Geometry check sheet. Reference: the model listing, model coordinates, mm. Face numbers are marked on the shaded views. A direction names the side the tool comes from. Round coordinates to 2 decimals unless told otherwise and drop trailing zeros. Order: outer loops, then holes, each group sorted by start corner. A loop starts at its lowest first (then second) coordinate and runs counter-clockwise, first axis right, second up. Notation, with made-up numbers: (73.5, 2.5) - (128.5, 2.5) arc R19 ccw to (128.5, 35.5) - close; hole circle Ø1 at (29, 42.5). An arc over 180 degrees is marked (long way). One line per question, with ' | ' between items. Start each with the question number.
Q1. Sectioned sample at B-B, the plane z = 12.5. Enter the section's corners in (x, y), then the cut area to 4 significant figures.
Q2. Gauge pin test, flat ends, axial feed: P1, Ø8, axis at x = 25, y = 17.5, coming from the -Z side; P2, Ø2.5, axis at x = 2, z = 25.5, coming from the +Y side; P3, Ø5, axis at x = 8, z = 18.5, coming from the +Y side; P4, Ø0.9, axis at x = 43.5, z = 16, coming from the +Y side. Record the tip position at first contact, or that the pin passes through.
Q3. Mould release check, pull along Z, two halves, no side actions. Record for the marked faces 3, 4, 5 and 6: +Z half, -Z half, draft (parallel to the pull), parting line (faces both ways), or undercut.
Q4. Sectioned sample at A-A, the plane y = 5.5. Enter the section's corners in (x, z).
Q5. Sectioned sample at C-C, the plane x = 7. Enter the section's corners in (y, z), then the cut area to 4 significant figures.
Q6. Sectioned sample at D-D, the plane z = 1. Enter the section's corners in (x, y).
Q7. Tool access check on the marked faces 1 and 2. Record the directions out of +Z, -Z, +X, -X, +Y, -Y that give a thin tool (end or side, any length) a straight path to the whole face; none if there is none.
Q8. Material ranges on line 1 along X through (y, z) = (12.5, 32.5); line 2 along X through (y, z) = (14.3, 16); line 3 along Z through (x, y) = (43, 15.3), recorded low to high.
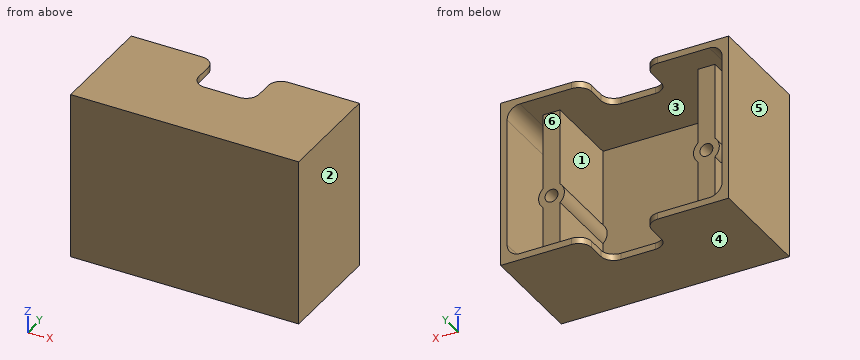
```python
from build123d import *

# Parameters (mm, degrees)
SKETCH1_W           = 50
SKETCH1_H           = 36
BOSS_EXTRUDE1_DEPTH = 24
SHELL1_T            = 1.5
SKETCH2_W           = 4
SKETCH2_H           = 36
BOSS_EXTRUDE2_DEPTH = 18
SKETCH6_W           = 14
SKETCH6_H           = 14
CUT_EXTRUDE2_DEPTH  = 58
FILLET1_R           = 3
SKETCH4_R           = 3
BOSS_EXTRUDE3_DEPTH = 18
SKETCH7_R           = 1.5
CUT_EXTRUDE3_DEPTH  = 5


with BuildPart() as part:
    # Sketch1 → Boss-Extrude1 (new body)
    with BuildSketch(Plane(origin=(0, 0, 0), x_dir=(1, 0, 0), z_dir=(0, 1, 0))):
        with Locations((25, -18)):
            Rectangle(SKETCH1_W, SKETCH1_H)
    extrude(amount=BOSS_EXTRUDE1_DEPTH)

    # Shell1
    shell1_openings = [part.faces().sort_by_distance(p)[0] for p in [
        (25, 24, 18),
    ]]
    offset(amount=SHELL1_T, openings=shell1_openings, kind=Kind.INTERSECTION)

    # Sketch2 → Boss-Extrude2 (add)
    with BuildSketch(Plane(origin=(0, 0, 0), x_dir=(1, 0, 0), z_dir=(0, 1, 0))):
        with Locations((7, -18)):
            Rectangle(SKETCH2_W, SKETCH2_H)
        with Locations((43, -18)):
            Rectangle(SKETCH2_W, SKETCH2_H)
    extrude(amount=BOSS_EXTRUDE2_DEPTH)

    # Sketch6 → Cut-Extrude2 (cut)
    with BuildSketch(Plane.XY.offset(37.5)):
        with Locations((25, 21.134691447)):
            Rectangle(SKETCH6_W, SKETCH6_H)
    extrude(amount=-CUT_EXTRUDE2_DEPTH, mode=Mode.SUBTRACT)

    # Fillet1
    fillet1_edges = [part.edges().sort_by_distance(p)[0] for p in [
        (0, 12, 0),
        (0, 12, 36),
        (50, 12, 36),
        (50, 12, 0),
        (32, 24, -0.75),
        (32, 24, 36.75),
        (18, 24, 36.75),
        (18, 24, -0.75),
        (32, 14.134691447, 36.75),
        (32, 14.134691447, -0.75),
        (18, 14.134691447, -0.75),
        (18, 14.134691447, 36.75),
    ]]
    fillet(fillet1_edges, radius=FILLET1_R)

    # Sketch4 → Boss-Extrude3 (add)
    with BuildSketch(Plane(origin=(0, 18, 0), x_dir=(1, 0, 0), z_dir=(0, 1, 0))):
        with Locations((7, -16)):
            Circle(SKETCH4_R)
        with Locations((43, -16)):
            Circle(SKETCH4_R)
    extrude(amount=-BOSS_EXTRUDE3_DEPTH)

    # Sketch7 → Cut-Extrude3 (cut)
    with BuildSketch(Plane(origin=(0, 18, 0), x_dir=(1, 0, 0), z_dir=(0, 1, 0))):
        with Locations(Location((7, -16, 0), (0, 0, 270))):
            Circle(SKETCH7_R)
        with Locations(Location((43, -16, 0), (0, 0, 90))):
            Circle(SKETCH7_R)
    extrude(amount=-CUT_EXTRUDE3_DEPTH, mode=Mode.SUBTRACT)


solid = part.part
```
Determined:
1) outline: (-1.5, -1.5) - (51.5, -1.5) - (51.5, 24) - (50, 24) - (50, 0) - (45, 0) - (45, 18) - (41, 18) - (41, 0) - (9, 0) - (9, 18) - (5, 18) - (5, 0) - (0, 0) - (0, 24) - (-1.5, 24) - close | area: 295.5 mm2
2) P1: stops at z = -1.5 | P2: stops at y = 0 | P3: stops at y = 18 | P4: stops at y = 13
3) face 3: undercut | face 4: -Z half | face 5: draft | face 6: undercut
4) outline: (-1.5, -1.5) - (51.5, -1.5) - (51.5, 37.5) - (-1.5, 37.5) - close; hole (0, 3) arc R3 ccw to (3, 0) - (5, 0) - (5, 13.76) arc R3 cw to (5, 18.24) - (5, 36) - (3, 36) arc R3 ccw to (0, 33) - close; hole (9, 0) - (41, 0) - (41, 13.76) arc R3 cw to (41, 18.24) - (41, 36) - (9, 36) - (9, 18.24) arc R3 cw to (9, 13.76) - close; hole (45, 0) - (47, 0) arc R3 ccw to (50, 3) - (50, 33) arc R3 ccw to (47, 36) - (45, 36) - (45, 18.24) arc R3 cw to (45, 13.76) - close
5) outline: (-1.5, -1.5) - (24, -1.5) - (24, 0) - (18, 0) - (18, 14.5) - (13, 14.5) - (13, 17.5) - (18, 17.5) - (18, 36) - (24, 36) - (24, 37.5) - (-1.5, 37.5) - close | area: 763.5 mm2
6) outline: (-1.5, -1.5) - (51.5, -1.5) - (51.5, 24) - (49.24, 24) - (49.24, 0) - (45, 0) - (45, 18) - (41, 18) - (41, 0) - (9, 0) - (9, 18) - (5, 18) - (5, 0) - (0.76, 0) - (0.76, 24) - (-1.5, 24) - close
7) face 1: +Y | face 2: +Z, -Z, +X, +Y, -Y
8) line 1: x = -1.5 to 0, 5 to 9, 41 to 45, 50 to 51.5 | line 2: x = -1.5 to 0, 4 to 5.5, 8.5 to 10, 40 to 41.5, 44.5 to 46, 50 to 51.5 | line 3: z = -1.5 to 14.5, 17.5 to 37.5
